Read the model definition and answer for the solid it produces. Units are mm, in the model's axes. A direction names the side the tool comes from. Coordinates: 2 decimals unless noted, no trailing zeros. Order: outer loops, then holes, each group sorted by start corner. A loop starts at its lowest first (then second) coordinate and runs counter-clockwise, first axis right, second up. Notation, with made-up numbers: M -37.75,-39 L 18.25,-39 A21 ccw 18.25,-1 Z; hole C 34.5,88 d10. An arc over 180 degrees is marked long. Write each question's results on one line, items separated by ' | '.
```python
from build123d import *

# Parameters (mm, degrees)
ESBO_O2_W             = 5.89486681
ESBO_O2_H             = 1
CORTE_EXTRUS_O1_DEPTH = 1


with BuildPart() as part:
    # Esboço1 → Revolução1 (revolve)
    with BuildSketch(Plane(origin=(0, 0, 0), x_dir=(1, 0, 0), z_dir=(0, 1, 0))):
        with BuildLine():
            Line((0, 0), (0, 1.5))
            Line((0, 1.5), (2.123676058, 1.5))
            ThreePointArc((2.123676058, 1.5), (2.478059498, 0.786906045), (2.6, 0))
            Line((2.6, 0), (1.425, 0))
            Line((1.425, 0), (1.425, -11.575))
            Line((1.425, -11.575), (0, -13))
            Line((0, -13), (0, 0))
        make_face()
    revolve(axis=Axis((0, 0, 0), (0, 0, 1)))

    # Esboço2 → Corte-extrusão1 (cut)
    with BuildSketch(Plane(origin=(0, 0, -1.5), x_dir=(-1, 0, 0), z_dir=(0, 0, -1))):
        Rectangle(ESBO_O2_W, ESBO_O2_H)
    extrude(amount=-CORTE_EXTRUS_O1_DEPTH, mode=Mode.SUBTRACT)


solid = part.part
```
(1) Given pin 1 (1 mm diameter, centred on x = 0, z = 4.5, fed in from -Y) (3 decimals); pin 2 (0.5 mm diameter, centred on x = 0.5, z = -1, fed in from -Y), each flat-ended and moving along its own axis, determine where each tip first touches the part or whether it passes through.
Conclusion:
pin 1: y = -1.425 | pin 2: y = -2.45
(2) The part is cut by section B-B, the plane y = -1.8. Write down the section's boundary in (x, z).
Conclusion:
outline: M -1.88,0 A1.88 ccw -1.13,-1.5 L 1.13,-1.5 A1.88 ccw 1.88,0 Z
(3) Straight lines are drawn through the part: line 1 (Z direction, x = -1.9, y = 0.6); line 2 (Y direction, x = -0.1, z = 1); line 3 (Z direction, x = 1.8, y = -0.45). For each, find the intervals that lie inside material, in ascending order.
Conclusion:
line 1: -1.5 to 0 | line 2: -1.42 to 1.42 | line 3: -0.5 to 0
(4) The part is cut by section A-A, the plane z = 8. Write down the section's boundary in (x, y) (3 decimals).
Conclusion:
outline: C 0,0 d2.85
(5) For faces 1 (the flat face through (0, -0.5, -1)), 2 (the conical face through (0, 0, 13)), determine the directions among +Z, -Z, +X, -X, +Y, -Y from which every point of the face is accessible in a straight line to the end or side of a thin tool.
Conclusion:
face 1: -Z, +X, -X | face 2: +Z
(6) The mould has two halves that part along Y. Classify faces 3 (the flat face through (1.12, -1.12, 0)), 4 (the flat face through (0, 0.5, -1)), 5 (the cylindrical face through (-1.13, -0.87, 5.87)): pulls with the +Y half, pulls with the -Y half, needs draft (parallel to the pull), parting line crosses it, or undercut.
Conclusion:
face 3: needs draft | face 4: undercut | face 5: parting line crosses it
